from build123d import *

# Parameters (mm, degrees)
SKETCH1_R                                      = 15.875
BOSS_EXTRUDE1_DEPTH                            = 7.62
SKETCH2_R                                      = 6.35
CUT_EXTRUDE1_DEPTH                             = 24.708556472
CIRPATTERN1_COUNT                              = 3
CBORE_FOR_6_SOCKET_HEAD_CAP_SCREW1_D           = 3.6576
CBORE_FOR_6_SOCKET_HEAD_CAP_SCREW1_CBORE_D     = 7.14502
CBORE_FOR_6_SOCKET_HEAD_CAP_SCREW1_CBORE_DEPTH = 3.5052
CIRPATTERN2_COUNT                              = 2
SKETCH42_R                                     = 2.286
CUT_EXTRUDE2_DEPTH                             = 7.62
CIRPATTERN3_COUNT                              = 2
CUT_EXTRUDE3_DEPTH                             = 24.70855664


with BuildPart() as part:
    # Sketch1 → Boss-Extrude1 (new body)
    with BuildSketch(Plane.XY):
        with Locations(Location((0, 0, 0), (0, 0, 180))):
            Circle(SKETCH1_R)
    extrude(amount=BOSS_EXTRUDE1_DEPTH)

    # Sketch2 → Cut-Extrude1 (cut, through all)
    with BuildSketch(Plane.XY.offset(7.62)):
        Circle(SKETCH2_R)
    extrude(amount=-CUT_EXTRUDE1_DEPTH, mode=Mode.SUBTRACT)

    # Sketch36 → Tap Drill for #8-32 Tap1 (revolve, cut)
    with BuildSketch(Plane(origin=(-0.450397279, -15.875, 3.175), x_dir=(0, 0, -1), z_dir=(1, 0, 0))):
        Polygon((0, 0), (0, 20.499292883), (1.7272, 19.05), (1.7272, 0), align=None)
    tap_drill_for_8_32_tap1 = revolve(axis=Axis((-0.450397279, -22.225, 3.175), (0, 1, 0)), mode=Mode.SUBTRACT)

    # CirPattern1: Tap Drill for #8-32 Tap1 ×3 about axis
    cirpattern1_axis = Axis((0, 0, 7.62), (0, 0, -1))
    for i in range(1, CIRPATTERN1_COUNT):
        add(tap_drill_for_8_32_tap1.rotate(cirpattern1_axis, i * 360 / CIRPATTERN1_COUNT), mode=Mode.SUBTRACT)

    # CBORE for #6 Socket Head Cap Screw1 (through all)
    with Locations(Plane(origin=(0, 0, 0), x_dir=(-1, 0, 0), z_dir=(0, 0, -1))):
        with Locations((4.769587089, -10.050926029)):
            cbore_for_6_socket_head_cap_screw1 = CounterBoreHole(CBORE_FOR_6_SOCKET_HEAD_CAP_SCREW1_D / 2, CBORE_FOR_6_SOCKET_HEAD_CAP_SCREW1_CBORE_D / 2, CBORE_FOR_6_SOCKET_HEAD_CAP_SCREW1_CBORE_DEPTH)

    # CirPattern2: CBORE for #6 Socket Head Cap Screw1 ×2 about axis
    cirpattern2_axis = Axis((0, 0, 0), (0, 0, 1))
    for i in range(1, CIRPATTERN2_COUNT):
        add(cbore_for_6_socket_head_cap_screw1.rotate(cirpattern2_axis, i * 360 / CIRPATTERN2_COUNT), mode=Mode.SUBTRACT)

    # Sketch42 → Cut-Extrude2 (cut)
    with BuildSketch(Plane(origin=(0, 0, 0), x_dir=(-1, 0, 0), z_dir=(0, 0, -1))):
        with Locations((4.365368762, 10.219159056)):
            Circle(SKETCH42_R)
    cut_extrude2 = extrude(amount=-CUT_EXTRUDE2_DEPTH, mode=Mode.SUBTRACT)

    # CirPattern3: Cut-Extrude2 ×2 about axis
    cirpattern3_axis = Axis((0, 0, 0), (0, 0, 1))
    for i in range(1, CIRPATTERN3_COUNT):
        add(cut_extrude2.rotate(cirpattern3_axis, i * 360 / CIRPATTERN3_COUNT), mode=Mode.SUBTRACT)

    # Sketch43 → Cut-Extrude3 (cut, through all)
    with BuildSketch(Plane(origin=(0, 0, 0), x_dir=(-1, 0, 0), z_dir=(0, 0, -1))):
        with BuildLine():
            Line((-8.025711128, -1.073137194), (-6.956985206, -3.563699487))
            ThreePointArc((-6.956985206, -3.563699487), (-7.355887027, -4.562271884), (-8.354459424, -4.163370063))
            Line((-8.354459424, -4.163370063), (-9.423185347, -1.67280777))
            ThreePointArc((-9.423185347, -1.67280777), (-9.024283525, -0.674235373), (-8.025711128, -1.073137194))
        make_face()
    extrude(amount=-CUT_EXTRUDE3_DEPTH, mode=Mode.SUBTRACT)


solid = part.part
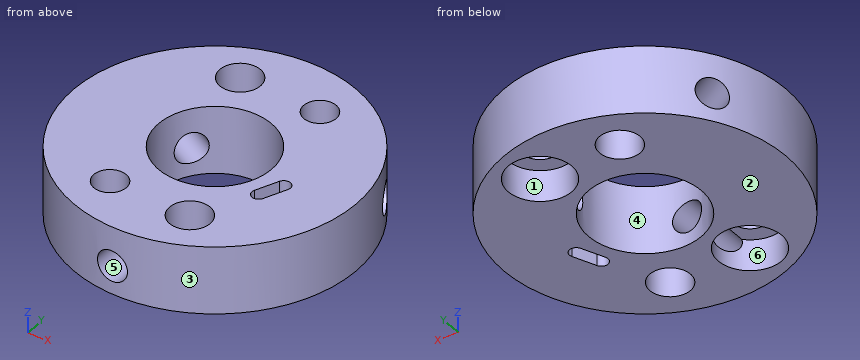
The listing builds one solid part. Answer for the finished solid, in the listing's coordinates (mm). Face numbers are marked on the shaded views. A direction names the side the tool comes from. Coordinates: 2 decimals unless noted, no trailing zeros. Order: outer loops, then holes, each group sorted by start corner. A loop starts at its lowest first (then second) coordinate and runs counter-clockwise, first axis right, second up. Notation, with made-up numbers: M -3.75,24 L 13.25,24 A17 ccw 13.25,30 Z; hole C 88,84 d11. An arc over 180 degrees is marked long. Use CSV: the item, a comma, the result in double quotes.
Q1. A tool of negligible diameter and unlimited length cuts with its end or side. For the marked faces 4, 5 and 6, from which of +Z, -Z, +X, -X, +Y, -Y can it reach the whole face along a straight path? Write none if from no direction.
Here are the results:
face 4,"+Z, -Z"
face 5,"-Y"
face 6,"-Z"
Q2. Given pin 1 Ø1 at (x, y) = (-6, -12.5) entering from -Z; pin 2 Ø4 at (x, z) = (-12.5, 4) entering from +Y, each flat-ended and moving along its own axis, determine where each tip first touches the part or whether it passes through.
Here are the results:
pin 1,"z = 3.51"
pin 2,"y = 11.91"
Q3. Section D-D (z = 5.5) is taken. Determine the outline of the cut face in (x, y) (3 decimals).
Here are the results:
outline,"C 0,0 d31.75; hole C -4.365,10.219 d4.572; hole C -4.77,-10.051 d3.658; hole C 0,0 d12.7; hole C 4.365,-10.219 d4.572; hole C 4.77,10.051 d3.658; hole M 6.957,-3.564 A0.76 ccw 8.354,-4.163 L 9.423,-1.673 A0.76 ccw 8.026,-1.073 Z"
Q4. Section A-A (y = 0) is taken. Determine the outline of the cut face in (x, z) (3 decimals).
Here are the results:
outline,"M -15.875,0 L -6.35,0 L -6.35,7.62 L -15.875,7.62 Z; M 6.35,0 L 15.875,0 L 15.875,7.62 L 6.35,7.62 Z"
Q5. Determine the mould class of the marked faces 1, 2 and 3 for opening direction X: pulls with the +X half, pulls with the -X half, needs draft (parallel to the pull), parting line crosses it, or undercut.
Here are the results:
face 1,"undercut"
face 2,"needs draft"
face 3,"parting line crosses it"
Q6. Section B-B (z = 3) is taken. Give the number of separate pieces and of enclosed holes in the cut face, then the cut area to 3 significant figures.
Here are the results:
separate pieces,"3"
enclosed holes,"4"
area,"451 mm2"
Q7. Section C-C (x = 0) is taken. Determine the outline of the cut face in (y, z) (3 decimals).
Here are the results:
outline,"M -15.875,0 L -6.35,0 L -6.35,1.508 L -15.875,1.508 Z; M -15.875,4.842 L -6.35,4.842 L -6.35,7.62 L -15.875,7.62 Z; M 6.35,0 L 15.875,0 L 15.875,7.62 L 6.35,7.62 Z"
Q8. Straight lines are drawn through the part: L1, parallel to X at y = -3, z = 2.5; L2, parallel to X at y = 5.5, z = 3; L3, parallel to Y at x = -3, z = 2.25. For each, find the intervals that lie inside material, in ascending order.
Here are the results:
L1,"-15.59 to -5.6, 5.6 to 7.2, 8.85 to 15.59"
L2,"-14.89 to -12.06, -5.19 to -3.17, 3.17 to 6.99, 13.86 to 14.89"
L3,"-15.59 to -13.15, -6.95 to -5.6, 5.6 to 8.39, 12.05 to 15.59"
